Read the model definition and answer for the solid it produces. Units are mm, in the model's axes. Face numbers are marked on the shaded views. A direction names the side the tool comes from. Round coordinates to 2 decimals unless told otherwise and drop trailing zeros. Order: outer loops, then holes, each group sorted by start corner. A loop starts at its lowest first (then second) coordinate and runs counter-clockwise, first axis right, second up.
from build123d import *

# Parameters (mm, degrees)
F0_R     = 2.265
F0_R_2   = 2
F0_R_3   = 14
F1_DEPTH = 8


with BuildPart() as f1:
    # F0 (on Top) → F1 (new body)
    with BuildSketch(Plane.XY):
        with BuildLine():
            Line((-88.381675, 1.503936), (-106.949748, 1.503936))
            ThreePointArc((-106.949748, 1.503936), (-110.485281, 0.03947), (-111.949748, -3.496064))
            Line((-111.949748, -3.496064), (-111.949748, -39.266064))
            ThreePointArc((-111.949748, -39.266064), (-110.485281, -42.801598), (-106.949748, -44.266064))
            Line((-106.949748, -44.266064), (-84.717208, -44.266064))
            Line((-84.717208, -44.266064), (-33.233784, -44.266064))
            ThreePointArc((-33.233784, -44.266064), (-29.69825, -42.801598), (-28.233784, -39.266064))
            Line((-28.233784, -39.266064), (-28.233784, -3.496064))
            ThreePointArc((-28.233784, -3.496064), (-29.69825, 0.03947), (-33.233784, 1.503936))
            Line((-33.233784, 1.503936), (-57.51782, 1.503936))
            ThreePointArc((-57.51782, 1.503936), (-57.830224, 1.553986), (-58.111356, 1.699128))
            ThreePointArc((-58.111356, 1.699128), (-72.949748, 6.578936), (-87.788139, 1.699128))
            ThreePointArc((-87.788139, 1.699128), (-88.069271, 1.553986), (-88.381675, 1.503936))
        make_face()
        with BuildLine():
            Line((-101.799748, -33.231064), (-101.799748, -38.381064))
            ThreePointArc((-101.799748, -38.381064), (-104.024748, -40.606064), (-106.249748, -38.381064))
            Line((-106.249748, -38.381064), (-106.249748, -33.231064))
            ThreePointArc((-106.249748, -33.231064), (-104.024748, -31.006064), (-101.799748, -33.231064))
        make_face(mode=Mode.SUBTRACT)
        with Locations((-86.384776, -31.856093)):
            Circle(F0_R, mode=Mode.SUBTRACT)
        with Locations((-59.514719, -31.856093)):
            Circle(F0_R, mode=Mode.SUBTRACT)
        with Locations((-51.721655, -38.381064)):
            Circle(F0_R_2, mode=Mode.SUBTRACT)
        with Locations((-35.233784, -38.381064)):
            Circle(F0_R_2, mode=Mode.SUBTRACT)
        with Locations((-72.949748, -18.421064)):
            Circle(F0_R_3, mode=Mode.SUBTRACT)
        with BuildLine():
            Line((-106.249748, -13.531064), (-106.249748, -8.381064))
            ThreePointArc((-106.249748, -8.381064), (-104.024748, -6.156064), (-101.799748, -8.381064))
            Line((-101.799748, -8.381064), (-101.799748, -13.531064))
            ThreePointArc((-101.799748, -13.531064), (-104.024748, -15.756064), (-106.249748, -13.531064))
        make_face(mode=Mode.SUBTRACT)
        with Locations((-86.384776, -4.986036)):
            Circle(F0_R, mode=Mode.SUBTRACT)
        with Locations((-59.514719, -4.986036)):
            Circle(F0_R, mode=Mode.SUBTRACT)
    extrude(amount=F1_DEPTH)


solid = f1.part
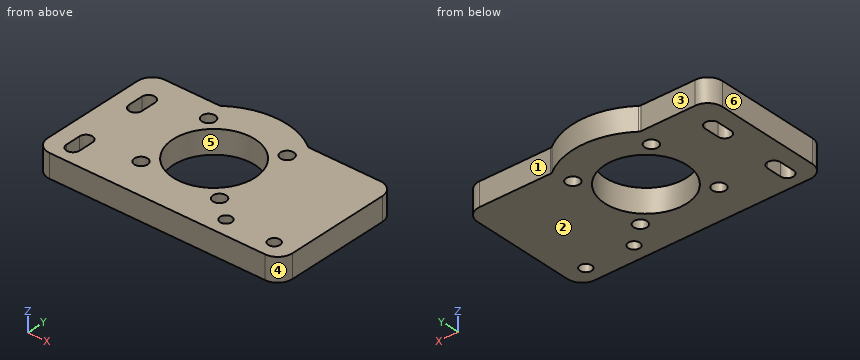
Q1. A cutting plane is placed at D-D, the plane x = -95. Give the vertices of the cut face in (y, z), plus the area to 3 significant figures.
Outcome:
outline: (-44.27, 0) - (1.5, 0) - (1.5, 8) - (-44.27, 8) - close
area: 366 mm2
Q2. Straight lines are drawn through the part: probe 1 along X at (y, z) = (-36, 4.25); probe 2 along X at (y, z) = (-37, 2.25); probe 3 along X at (y, z) = (-37.5, 7.25). For each, find the intervals that lie inside material, in ascending order.
Outcome:
probe 1: x = -111.95 to -106.25, -101.8 to -28.23
probe 2: x = -111.95 to -106.25, -101.8 to -53.17, -50.28 to -36.68, -33.79 to -28.23
probe 3: x = -111.95 to -106.25, -101.8 to -53.52, -49.93 to -37.03, -33.44 to -28.23
Q3. A cutting plane is placed at C-C, the plane z = 1.5. Give the number of separate pieces and of enclosed holes in the cut face, plus the area to 3 significant figures.
Outcome:
separate pieces: 1
enclosed holes: 9
area: 3,130 mm2
Q4. A flat-ended cylindrical pin translates along its axis: pin 1 (1.5 mm diameter, centred on x = -97.5, z = 1, fed in from +Y). Find the tip coordinate at first contact, or state that the pin passes through.
Outcome:
pin 1: stops at y = 1.5
Q5. For a pull along Y with two mould halves and no side action, classify the marked faces 4, 5 and 6 as released by +Y, released by -Y, zero draft, split by the parting line, or undercut.
Outcome:
face 4: released by -Y
face 5: undercut
face 6: zero draft
Q6. For the marked faces 1, 2 and 3, determine the directions among +Z, -Z, +X, -X, +Y, -Y from which every point of the face is accessible in a straight line to the end or side of a thin tool.
Outcome:
face 1: +Z, -Z, +X, +Y
face 2: -Z, +X, -X, +Y, -Y
face 3: +Z, -Z, -X, +Y
Q7. A cutting plane is placed at A-A, the plane x = -65.5. Give the vertices of the cut face in (y, z).
Outcome:
outline: (-44.27, 0) - (-30.27, 0) - (-30.27, 8) - (-44.27, 8) - close; (-6.57, 0) - (5.44, 0) - (5.44, 8) - (-6.57, 8) - close
Q8. A cutting plane is placed at B-B, the plane y = -24.5. Give the vertices of the cut face in (x, z), plus the area to 3 significant figures.
Outcome:
outline: (-111.95, 0) - (-85.56, 0) - (-85.56, 8) - (-111.95, 8) - close; (-60.34, 0) - (-28.23, 0) - (-28.23, 8) - (-60.34, 8) - close
area: 468 mm2
